```python
from build123d import *

# Parameters (mm, degrees)
BOSS_EXTRUDE4_DEPTH = 3
SKETCH10_W          = 6
SKETCH10_H          = 42.3
BOSS_EXTRUDE5_DEPTH = 3
SKETCH11_R          = 12
SKETCH11_R_2        = 1.6
CUT_EXTRUDE1_DEPTH  = 7
SKETCH15_W          = 3
SKETCH15_H          = 42.3
BOSS_EXTRUDE8_DEPTH = 20
FILLET5_R           = 1
SKETCH16_R          = 3.4
CUT_EXTRUDE5_DEPTH  = 4
SKETCH23_W          = 20
SKETCH23_H          = 42.3
BOSS_EXTRUDE9_DEPTH = 3
SKETCH26_W          = 12.4
SKETCH26_H          = 13.3
CUT_EXTRUDE7_DEPTH  = 3


with BuildPart() as part:
    # Sketch3 → Boss-Extrude4 (new body)
    with BuildSketch(Plane.XY):
        Polygon((0, 0), (42.3, 0), (42.3, 42.3), (0, 42.3), (-4, 42.3), (-4, 0), align=None)
    extrude(amount=BOSS_EXTRUDE4_DEPTH)

    # Sketch10 → Boss-Extrude5 (add)
    with BuildSketch(Plane.ZY.offset(4)):
        with Locations((0, 21.15)):
            Rectangle(SKETCH10_W, SKETCH10_H)
    extrude(amount=BOSS_EXTRUDE5_DEPTH)

    # Sketch11 → Cut-Extrude1 (cut, through all)
    with BuildSketch(Plane.XY.offset(3)):
        with Locations((21.65, 21.15)):
            Circle(SKETCH11_R)
        with Locations((6.15, 36.65)):
            Circle(SKETCH11_R_2)
        with Locations((37.15, 36.65)):
            Circle(SKETCH11_R_2)
        with Locations((37.15, 5.65)):
            Circle(SKETCH11_R_2)
        with Locations((6.15, 5.65)):
            Circle(SKETCH11_R_2)
    extrude(amount=-CUT_EXTRUDE1_DEPTH, mode=Mode.SUBTRACT)

    # Sketch15 → Boss-Extrude8 (add)
    with BuildSketch(Plane.ZY.offset(7)):
        with Locations((1.5, 21.15)):
            Rectangle(SKETCH15_W, SKETCH15_H)
    extrude(amount=BOSS_EXTRUDE8_DEPTH)

    # Fillet5
    fillet5_edges = [part.edges().sort_by_distance(p)[0] for p in [
        (42.3, 0, 1.5),
        (42.3, 42.3, 1.5),
    ]]
    fillet(fillet5_edges, radius=FILLET5_R)

    # Sketch16 → Cut-Extrude5 (cut, through all)
    with BuildSketch(Plane(origin=(0, 0, 0), x_dir=(-1, 0, 0), z_dir=(0, 0, -1))):
        with Locations((17.55, 21.15)):
            Circle(SKETCH16_R)
    extrude(amount=-CUT_EXTRUDE5_DEPTH, mode=Mode.SUBTRACT)

    # Sketch23 → Boss-Extrude9 (add)
    with BuildSketch(Plane(origin=(0, 0, 0), x_dir=(-1, 0, 0), z_dir=(0, 0, -1))):
        with Locations((17, 21.15)):
            Rectangle(SKETCH23_W, SKETCH23_H)
    extrude(amount=BOSS_EXTRUDE9_DEPTH)

    # Sketch26 → Cut-Extrude7 (cut)
    with BuildSketch(Plane(origin=(0, 0, -3), x_dir=(-1, 0, 0), z_dir=(0, 0, -1))):
        with Locations((17.55, 21.15)):
            Rectangle(SKETCH26_W, SKETCH26_H)
    extrude(amount=-CUT_EXTRUDE7_DEPTH, mode=Mode.SUBTRACT)


solid = part.part
```
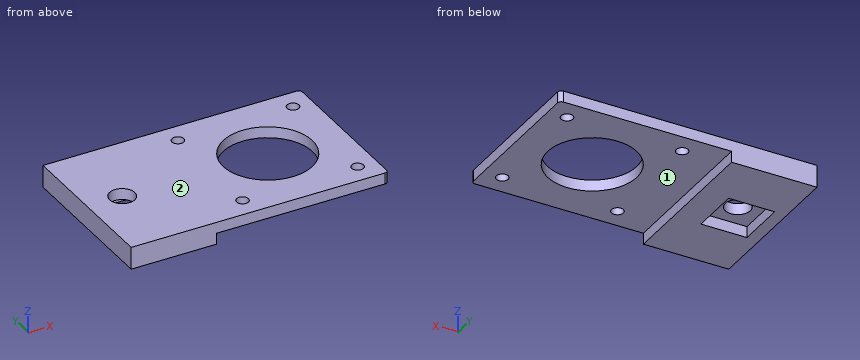
Geometry: final body of the model. Coordinates: model frame, mm. Face numbers are marked on the shaded views. A direction names the side the tool comes from. Coordinates: 2 decimals unless noted, no trailing zeros. Order: outer loops, then holes, each group sorted by start corner. A loop starts at its lowest first (then second) coordinate and runs counter-clockwise, first axis right, second up.
Item 1: Section query B-B (x = 37.15). Output: boundary loops of the cut face in (y, z).
Answer:
outline: (0, 0) - (4.05, 0) - (4.05, 3) - (0, 3) - close; (7.25, 0) - (35.05, 0) - (35.05, 3) - (7.25, 3) - close; (38.25, 0) - (42.3, 0) - (42.3, 3) - (38.25, 3) - close
Item 2: Contact query for flat-ended pins moving along their axis: P1, Ø1.5, axis at y = 24, z = -1.5, coming from the +X side; P2, Ø13.5, axis at x = -17, y = 18, coming from the -Z side. Output: stop coordinate, or through.
Answer:
P1: stops at x = -4
P2: stops at z = -3
Item 3: Section query A-A (y = 21.15). Output: boundary loops of the cut face in (x, z).
Answer:
outline: (-27, -3) - (-23.75, -3) - (-23.75, 0) - (-20.95, 0) - (-20.95, 3) - (-27, 3) - close; (-14.15, 0) - (-11.35, 0) - (-11.35, -3) - (-4, -3) - (-4, 0) - (9.65, 0) - (9.65, 3) - (-14.15, 3) - close; (33.65, 0) - (42.3, 0) - (42.3, 3) - (33.65, 3) - close
Item 4: Access query for the marked faces 1 and 2. Directions: +Z, -Z, +X, -X, +Y, -Y. A direction counts if a zero-diameter tool reaches every point of the face in a straight line with its end or side. Return the directions, or none.
Answer:
face 1: -Z, +X, +Y, -Y
face 2: +Z, +X, -X, +Y, -Y
Item 5: Material intervals for line 1 along Y through (x, z) = (37.15, 2.2); line 2 along Y through (x, z) = (21.65, 2); line 3 along Y through (x, z) = (-13, -1.5), sorted ascending.
Answer:
line 1: y = 0 to 4.05, 7.25 to 35.05, 38.25 to 42.3
line 2: y = 0 to 9.15, 33.15 to 42.3
line 3: y = 0 to 14.5, 27.8 to 42.3
Item 6: Section query C-C (z = 1). Output: boundary loops of the cut face in (x, y), then the cut area to 3 significant figures.
Answer:
outline: (-27, 0) - (41.3, 0) arc R1 ccw to (42.3, 1) - (42.3, 41.3) arc R1 ccw to (41.3, 42.3) - (-27, 42.3) - close; hole circle Ø6.8 at (-17.55, 21.15); hole circle Ø3.2 at (6.15, 5.65); hole circle Ø3.2 at (6.15, 36.65); hole circle Ø24 at (21.65, 21.15); hole circle Ø3.2 at (37.15, 5.65); hole circle Ø3.2 at (37.15, 36.65)
area: 2,410 mm2
Item 7: Section query D-D (x = -17.55). Output: boundary loops of the cut face in (y, z).
Answer:
outline: (0, -3) - (14.5, -3) - (14.5, 0) - (17.75, 0) - (17.75, 3) - (0, 3) - close; (24.55, 0) - (27.8, 0) - (27.8, -3) - (42.3, -3) - (42.3, 3) - (24.55, 3) - close
